Can you work these out from the model? Positions are in its coordinate system, mm. Round coordinates to 2 decimals unless told otherwise and drop trailing zeros. Loops run counter-clockwise (first coordinate to the right, second up) from the corner with the lowest first, then second, coordinate; pieces in that order, holes last. Notation, with made-up numbers: (-30.75, 43.5) -> (-8.75, 43.5) arc R28 ccw to (-8.75, 74.5) -> close; hole circle Ø7 at (-9.75, -34.5). An arc over 180 degrees is marked (long way). Write each question's results on one line, items separated by ' | '.
Autodesk Inventor part; units mm, degrees
ref_plane "YZ Plane" through (0, 0, 0) normal (1, 0, 0) x (0, 1, 0)
ref_plane "XZ Plane" through (0, 0, 0) normal (0, 1, 0) x (-1, 0, 0)
ref_plane "XY Plane" through (0, 0, 0) normal (0, 0, 1) x (1, 0, 0)
sketch "Sketch1" plane through (0, 0, 0) normal (0, 1, 0) x (-1, 0, 0)
  line L0 (-800, 1000) -> (800, 1000)
  line L1 (800, 1000) -> (800, -1000)
  line L2 (800, -1000) -> (-800, -1000)
  line L3 (-800, -1000) -> (-800, 1000)
  line L4 (-800, 1000) -> (800, -1000) construction
  line L5 (800, 1000) -> (-800, -1000) construction
  point P0 (0, 0)
  dimension "d0" = 2000
  dimension "d1" = 1600
extrude "Extrusion1" add sketch "Sketch1" along normal blind 12
sketch "Sketch2" plane through (0, 12, 0) normal (0, 1, 0) x (1, 0, 0)
  line L0 (-800, 1000) -> (-800, -1000) construction
  line L1 (-800, -1000) -> (800, -1000) construction
  line L2 (800, -1000) -> (800, 1000) construction
  line L3 (800, 1000) -> (-800, 1000) construction
  line L4 (-795, -995) -> (-795, 995)
  line L5 (-795, 995) -> (795, 995)
  line L6 (795, 995) -> (795, -995)
  line L7 (795, -995) -> (-795, -995)
  point P0 (0, 0)
  dimension "d4" = 5
extrude "Extrusion2" cut sketch "Sketch2" against normal blind 10
properties part number "stol_1"
1. If we section it at C-C (z = -579): List the corners of the cut face in (x, y) for me, then the cut area to 3 significant figures.
Final values:
outline: (-800, 0) -> (800, 0) -> (800, 12) -> (795, 12) -> (795, 2) -> (-795, 2) -> (-795, 12) -> (-800, 12) -> close | area: 3,300 mm2
2. Will this pin go through, and if not, where does the flat tip stop? pin 1 (10 mm diameter, centred on x = -444.5, z = 680.5, fed in from +Y).
Final values:
pin 1: y = 2
3. We'd pull the mould along X, two halves only. Please class faces 1 (the face through (11, 0, 14)), 2 (the face through (-11, 2, -14)): pulls with the +X half, pulls with the -X half, needs draft (parallel to the pull), parting line crosses it, or undercut.
Final values:
face 1: needs draft | face 2: undercut
4. Please list where these lines run through material, in increasing order: line 1 (Z direction, x = 78.5, y = 6.5); line 2 (X direction, y = 10.75, z = -482); line 3 (Y direction, x = -677, z = -444). Write a range as from..to.
Final values:
line 1: -1000..-995, 995..1000 | line 2: -800..-795, 795..800 | line 3: 0..2
5. If we section it at A-A (y = 4.75): List the corners of the cut face in (x, z) for me.
Final values:
outline: (-800, -1000) -> (800, -1000) -> (800, 1000) -> (-800, 1000) -> close; hole (-795, -995) -> (795, -995) -> (795, 995) -> (-795, 995) -> close
6. If we section it at B-B (x = -666.5): List the corners of the cut face in (y, z) for me.
Final values:
outline: (0, -1000) -> (12, -1000) -> (12, -995) -> (2, -995) -> (2, 995) -> (12, 995) -> (12, 1000) -> (0, 1000) -> close
